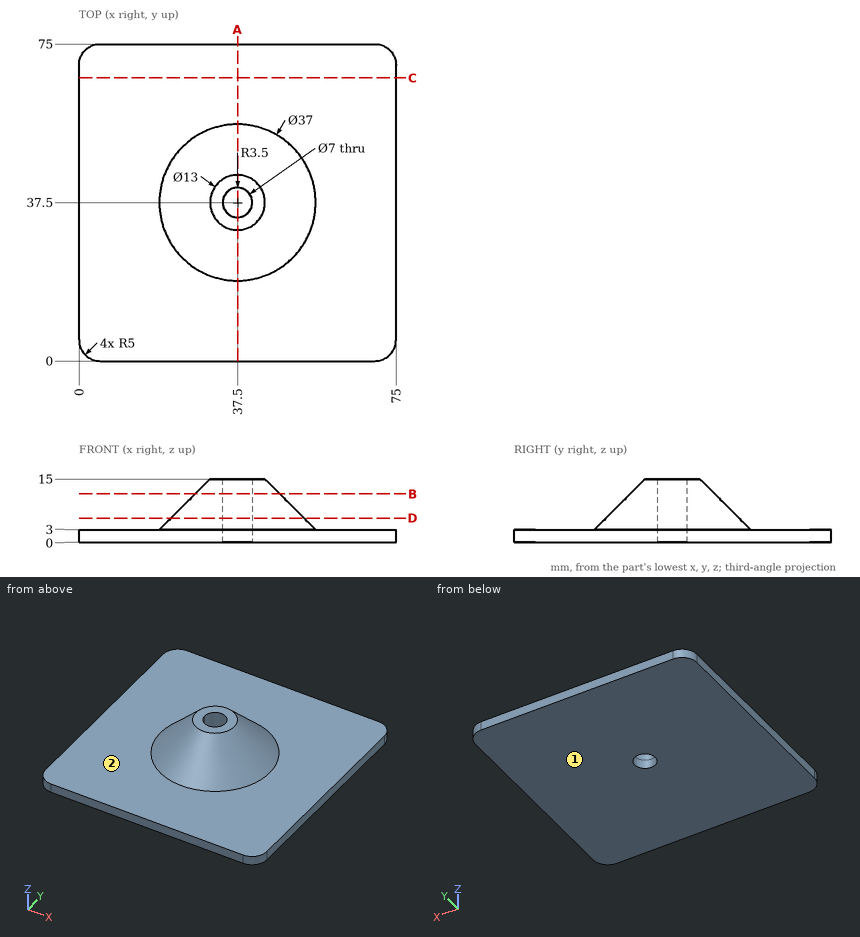
Here's the drawing with two shaded views (mm, measured from the low corner). I have some questions. A direction names the side the tool comes from. Give positions to 0.01 mm unless a question says otherwise; leave off trailing zeros. Write each loop counter-clockwise with the first axis right and the second up, starting at its lowest first coordinate (ties: lowest second). Pieces come first, ordered by that corner, then holes. Notation, with made-up numbers: (-31.75, 22) -> (-25.75, 22) arc R25 cw to (-25.75, 34) -> close; hole circle Ø5 at (53, -29). An arc over 180 degrees is marked (long way). Use one line per item in the form item = value.
1) Suppose I cut it at B-B (z = 11.5). Please give me the cut outline in (x, y), and give its area (3 significant figures).
Verdict:
outline = circle Ø20 at (37.5, 37.5); hole circle Ø7 at (37.5, 37.5)
area = 276 mm2
2) Suppose I cut it at D-D (z = 5.75). Please give me the cut outline in (x, y).
Verdict:
outline = circle Ø31.5 at (37.5, 37.5); hole circle Ø7 at (37.5, 37.5)
3) Suppose I cut it at C-C (y = 67). Please give me the cut outline in (x, z).
Verdict:
outline = (0, 0) -> (75, 0) -> (75, 3) -> (0, 3) -> close
4) I'm going to push a flat-ended pin straight in: pin 1 (5 mm diameter, centred on x = 8.5, y = 58, fed in from +Z). Where does the tip first touch, or does it pass through?
Verdict:
pin_1 = 3
5) If I drill on L1, parallel to Y at x = 37.5, z = 1.85; L2, parallel to Z at x = 4, y = 45.5, over which ranges is the centre line in solid material (lowest first)? Write a range as [from, to].
Verdict:
L1 = [0, 34], [41, 75]
L2 = [0, 3]
6) Suppose I cut it at A-A (x = 37.5). Please give me the cut outline in (y, z), and give its area (3 significant figures).
Verdict:
outline = (0, 0) -> (34, 0) -> (34, 15) -> (31, 15) -> (19, 3) -> (0, 3) -> close; (41, 0) -> (75, 0) -> (75, 3) -> (56, 3) -> (44, 15) -> (41, 15) -> close
area = 420 mm2
7) On a 3-axis mill with a long thin cutter (end or side, diameter ignored), from which of +Z, -Z, +X, -X, +Y, -Y can I reach the whole of each face in a straight line? I mean the marked faces 1 and 2. Say none if no direction works.
Verdict:
face_1 = -Z, +X, -X, +Y, -Y
face_2 = +Z
